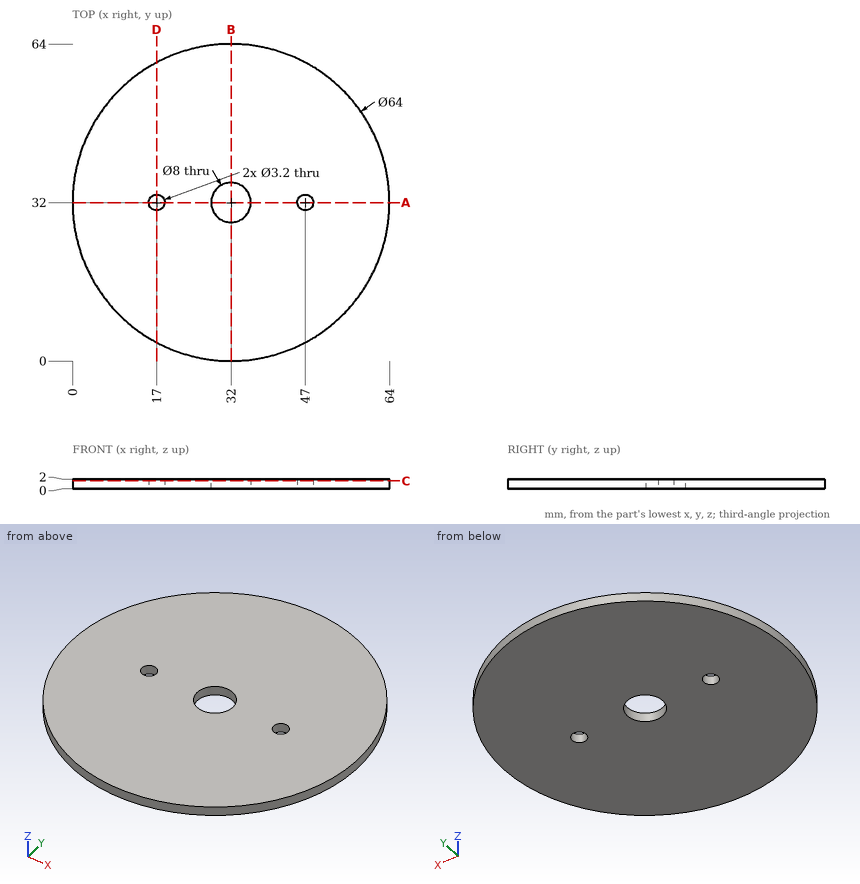
Source: three-view drawing plus pictorial views. Frame: mm from the lowest corner of the part. Coordinates: 2 decimals unless noted, no trailing zeros. Loops run counter-clockwise (first coordinate to the right, second up) from the corner with the lowest first, then second, coordinate; pieces in that order, holes last. Notation, with made-up numbers: (75, 28.25) - (122, 28.25) arc R36 cw to (122, 67.25) - close; hole circle Ø6 at (65, 2). An arc over 180 degrees is marked (long way). One line per item, written item: value. Start each with the question number.
1. Contact query for flat-ended pins moving along their axis: P1, Ø1, axis at x = 10, z = 0.5, coming from the -Y side; P2, Ø4, axis at x = 47, y = 32, coming from the -Z side; P3, Ø6.5, axis at x = 32, y = 32, coming from the -Z side. Output: stop coordinate, or through.
2. Section A-A (y = 32). Return the cut outline in (x, z), and give its area (3 significant figures).
3. Ray query, L1, parallel to Y at x = 32, z = 0.85; L2, parallel to Y at x = 30, z = 0.1; L3, parallel to X at y = 28.5, z = 0.3. Return the intervals inside material, ascending.
4. Section C-C (z = 1.6). Return the cut outline in (x, y), and give its area (3 significant figures).
5. Section B-B (x = 32). Return the cut outline in (y, z), and give its area (3 significant figures).
6. Section D-D (x = 17). Return the cut outline in (y, z).
Verdict:
1. P1: stops at y = 8.3
1. P2: stops at z = 0
1. P3: passes through
2. outline: (0, 0) - (15.4, 0) - (15.4, 2) - (0, 2) - close; (18.6, 0) - (28, 0) - (28, 2) - (18.6, 2) - close; (36, 0) - (45.4, 0) - (45.4, 2) - (36, 2) - close; (48.6, 0) - (64, 0) - (64, 2) - (48.6, 2) - close
2. area: 99.2 mm2
3. L1: y = 0 to 28, 36 to 64
3. L2: y = 0.06 to 28.54, 35.46 to 63.94
3. L3: x = 0.19 to 30.06, 33.94 to 63.81
4. outline: circle Ø64 at (32, 32); hole circle Ø3.2 at (17, 32); hole circle Ø8 at (32, 32); hole circle Ø3.2 at (47, 32)
4. area: 3,150 mm2
5. outline: (0, 0) - (28, 0) - (28, 2) - (0, 2) - close; (36, 0) - (64, 0) - (64, 2) - (36, 2) - close
5. area: 112 mm2
6. outline: (3.73, 0) - (30.4, 0) - (30.4, 2) - (3.73, 2) - close; (33.6, 0) - (60.27, 0) - (60.27, 2) - (33.6, 2) - close
